Here's how the part is built. I have some questions about the finished solid (model axes, mm). Face numbers are marked on the shaded views. A direction names the side the tool comes from. Coordinates: 2 decimals unless noted, no trailing zeros. Write each loop counter-clockwise with the first axis right and the second up, starting at its lowest first coordinate (ties: lowest second). Pieces come first, ordered by that corner, then holes.
```python
from build123d import *


with BuildPart() as part:
    # Эскиз1 → Повернуть1 (revolve)
    with BuildSketch(Plane.XZ, mode=Mode.PRIVATE) as revolve_1_sk:
        Polygon((11.7, 16.8), (13, 16.8), (13, 25.292893219), (12.292893219, 26), (10, 26), (10, 1), (11, 0), (12.5, 0), (13, 0.5), (13, 7.7), (11.7, 7.7), (11.7, 9), (15.5, 9), (15.5, 15), (11.7, 15), align=None)
    revolve(revolve_1_sk.sketch.rotate(Axis((0, 0, 26.005), (0, 0, -1)), 180), axis=Axis((0, 0, 26.005), (0, 0, -1)))


solid = part.part
```
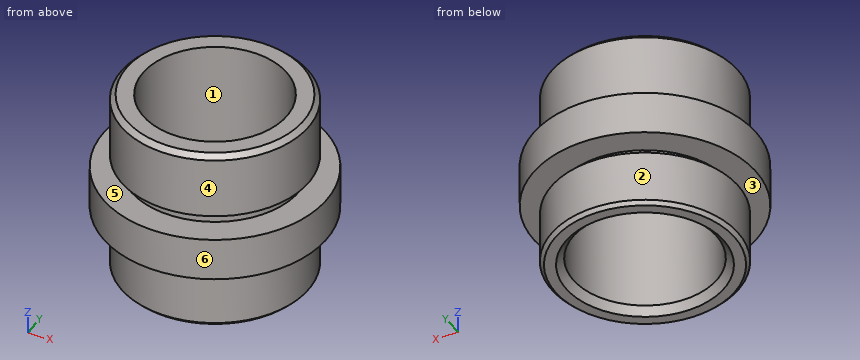
1) We'd pull the mould along Y, two halves only. Please class the marked faces 1, 2 and 3: pulls with the +Y half, pulls with the -Y half, needs draft (parallel to the pull), parting line crosses it, or undercut.
Values follow:
face 1: undercut
face 2: parting line crosses it
face 3: needs draft
2) Imagine slicing it at C-C on z = 19.5. Please give me the cut outline in (x, y), then the cut area to 3 significant figures.
Values follow:
outline: circle Ø26 at (0, 0); hole circle Ø20 at (0, 0)
area: 217 mm2
3) Imagine slicing it at D-D on z = 16.25. Please give me the cut outline in (x, y).
Values follow:
outline: circle Ø23.4 at (0, 0); hole circle Ø20 at (0, 0)
4) I need wall thicknesses on probe 1 along Y at (x, z) = (0, 14.75); probe 2 along Y at (x, z) = (2.5, 19.75); probe 3 along Z at (x, y) = (-12.5, -2.5). Which ranges of each line are inside material? Lowest first, please.
Values follow:
probe 1: y = -15.5 to -10, 10 to 15.5
probe 2: y = -12.76 to -9.68, 9.68 to 12.76
probe 3: z = 0.25 to 7.7, 9 to 15, 16.8 to 25.55
5) On a 3-axis mill with a long thin cutter (end or side, diameter ignored), from which of +Z, -Z, +X, -X, +Y, -Y can I reach the whole of each face in a straight line? I mean the marked faces 4, 5 and 6. Say none if no direction works.
Values follow:
face 4: +Z
face 5: none
face 6: +Z, -Z
6) Will these pins go through, and if not, where does the flat tip stop? pin 1 (4 mm diameter, centred on x = 11, z = 12.5, fed in from -Y); pin 2 (10 mm diameter, centred on y = -8.5, z = 15.5, fed in from -X); pin 3 (4 mm diameter, centred on x = 11, z = 18.5, fed in from +Y); pin 4 (16 mm diameter, centred on x = 0, y = 0, fed in from -Z).
Values follow:
pin 1: stops at y = -12.62
pin 2: stops at x = -15.09
pin 3: stops at y = 9.38
pin 4: passes through
